Work out the finished part from the listing and answer in its coordinate system (mm). A direction names the side the tool comes from. Round coordinates to 2 decimals unless told otherwise and drop trailing zeros. Write each loop counter-clockwise with the first axis right and the second up, starting at its lowest first coordinate (ties: lowest second). Pieces come first, ordered by that corner, then holes.
from build123d import *

# Parameters (mm, degrees)
F0_R     = 15
F1_DEPTH = 3
F2_R     = 2
F2_R_2   = 0.5
F3_DEPTH = 1.5
F4_R     = 2.5
F4_R_2   = 1.075
F5_DEPTH = 3


with BuildPart() as f1:
    # F0 (on Top) → F1 (new body)
    with BuildSketch(Plane.XY):
        with Locations((-16.1491949111, 10.887096636)):
            Circle(F0_R)
    extrude(amount=F1_DEPTH)

    # F2 (on face) → F3 (join)
    with BuildSketch(Plane.XY.offset(3)):
        with Locations((-12, 17.6008082926)):
            Circle(F2_R)
        with Locations((-12, 17.6008082926)):
            Circle(F2_R_2, mode=Mode.SUBTRACT)
        with BuildLine():
            ThreePointArc((-8.8824603224, 7.1392940688), (-16.7881056428, 5.1821903468), (-24.6329733241, 7.3702337589))
            ThreePointArc((-24.6329733241, 7.3702337589), (-19.4510459053, 3.8110892822), (-13.1690173954, 4.0477303202))
            add(Edge.make_bspline(
                [(-13.1690173954, 4.0477303202), (-13.1362154253, -1.1413398729), (-10.427309312, 0.097086679), (-7.7184031986, 1.335513231), (-11.8713523396, 4.6409819109)],
                knots=[3.8341028208, 3.8341028208, 3.8341028208, 6.2689537824, 6.2689537824, 8.7038047441, 8.7038047441, 8.7038047441], degree=2, weights=[1, 0.3460623341, 1, 0.3460623341, 1]))
            ThreePointArc((-11.8713523396, 4.6409819109), (-10.254077445, 5.743189869), (-8.8824603224, 7.1392940688))
        make_face()
        with BuildLine():
            ThreePointArc((-24.7671979005, 18.6823099732), (-22.0677226207, 18.8845619079), (-19.5026847059, 18.0193144708))
            ThreePointArc((-19.5026847059, 18.0193144708), (-21.9828567976, 19.558438644), (-24.7671979005, 18.6823099732))
        make_face()
    extrude(amount=F3_DEPTH)

    # F4 (on face) → F5 (join)
    with BuildSketch(Plane.XY.offset(3)):
        with Locations((-16.757108611, 27.0656452758)):
            Circle(F4_R)
        with Locations((-16.757108611, 27.0656452758)):
            Circle(F4_R_2, mode=Mode.SUBTRACT)
    extrude(amount=-F5_DEPTH)


solid = f1.part
Q1. Find section C-C (x = -20.5). Determine the outline of the cut face in (y, z).
Q2. A tool of negligible diameter and unlimited length cuts with its end or side. For faces 1 (the face through (-22.11, 18.89, 3.74)), 2 (the face through (-16.99, 26.016, 1.521)), from which of +Z, -Z, +X, -X, +Y, -Y can it reach the whole face along a straight path? Write none if from no direction.
Q3. Find section D-D (y = 22.5). Determine the outline of the cut face in (x, z), plus the area to 3 significant figures.
Q4. Find section B-B (z = 0.5). Determine the outline of the cut face in (x, y) (3 decimals), plus the area to 3 significant figures.
Q5. The mould has two halves that part along Y. Classify faces 3 (the face through (-21.941, 19.553, 3.74)), 4 (the face through (-16, 4, 4.5)), 5 (the face through (-16, 13, 3)): +Y half, -Y half, draft (parallel to the pull), parting line (faces both ways), or undercut.
Q6. Given pin 1 (2.5 mm diameter, centred on x = -16.76, y = 27.07, fed in from +Z), flat-ended and moving along its own axis, determine where the tip first touches the part or whether it passes through.
Q7. Find section A-A (y = 16.5). Determine the outline of the cut face in (x, z).
Q8. Find the intervals of material crossed by L1, parallel to Y at x = -12, z = 3.85; L2, parallel to Z at x = -15, y = 19.5; L3, parallel to Y at x = -16.5, z = 1.8, in increasing order.
Report:
1. outline: (-3.47, 0) - (25.24, 0) - (25.24, 3) - (19.01, 3) - (19.01, 4.5) - (18.49, 4.5) - (18.49, 3) - (5.67, 3) - (5.67, 4.5) - (4.18, 4.5) - (4.18, 3) - (-3.47, 3) - close
2. face 1: +Z
2. face 2: +Z, -Z
3. outline: (-25.64, 0) - (-6.65, 0) - (-6.65, 3) - (-25.64, 3) - close
3. area: 57.0 mm2
4. outline: (-18.816, 25.648) arc R15 ccw (long way) to (-14.597, 25.807) arc R2.5 ccw (long way) to start; hole circle Ø2.15 at (-16.757, 27.066)
4. area: 719 mm2
5. face 3: +Y half
5. face 4: draft
5. face 5: undercut
6. pin 1: stops at z = 3
7. outline: (-30.06, 0) - (-2.24, 0) - (-2.24, 3) - (-10.33, 3) - (-10.33, 4.5) - (-13.67, 4.5) - (-13.67, 3) - (-30.06, 3) - close
8. L1: y = 1.05 to 5.84, 15.6 to 17.1, 18.1 to 19.6
8. L2: z = 0 to 3
8. L3: y = -4.11 to 26.02, 28.11 to 29.55
